from build123d import *

# Parameters (mm, degrees)
SKETCH_2_W      = 30
SKETCH_2_H      = 30
EXTRUDE_1_DEPTH = 113
EXTRUDE_2_DEPTH = 15
SKETCH_4_W      = 30
SKETCH_4_H      = 20
EXTRUDE_4_DEPTH = 3


with BuildPart() as part:
    # 草图2 → 凸台-拉伸1 (new body)
    with BuildSketch(Plane(origin=(0, 0, 0), x_dir=(1, 0, 0), z_dir=(0, 1, 0))):
        with Locations((15, 15)):
            Rectangle(SKETCH_2_W, SKETCH_2_H)
    extrude(amount=EXTRUDE_1_DEPTH)

    # 草图3 → 凸台-拉伸2 (add)
    with BuildSketch(Plane.ZY):
        with BuildLine():
            Line((-30, 113), (-24.666190379, 113))
            ThreePointArc((-24.666190379, 113), (-25.206716397, 113.665063392), (-25.4, 114.5))
            Line((-25.4, 114.5), (-25.4, 119.8))
            Line((-25.4, 119.8), (-24.9, 119.8))
            Line((-24.9, 119.8), (-24.9, 120.3))
            Line((-24.9, 120.3), (-23.1, 120.3))
            Line((-23.1, 120.3), (-23.1, 117.9))
            Line((-23.1, 117.9), (-21.815685425, 117.9))
            Line((-21.815685425, 117.9), (-19.3, 120.415685425))
            Line((-19.3, 120.415685425), (-19.3, 125.584314575))
            Line((-19.3, 125.584314575), (-21.815685425, 128.1))
            Line((-21.815685425, 128.1), (-23.1, 128.1))
            Line((-23.1, 128.1), (-23.1, 125.7))
            Line((-23.1, 125.7), (-24.9, 125.7))
            Line((-24.9, 125.7), (-24.9, 126.2))
            Line((-24.9, 126.2), (-25.4, 126.2))
            Line((-25.4, 126.2), (-25.4, 131.5))
            ThreePointArc((-25.4, 131.5), (-25.206716397, 132.334936608), (-24.666190379, 133))
            Line((-24.666190379, 133), (-30, 133))
            Line((-30, 133), (-30, 113))
        make_face()
        Polygon((-18.2, 113.1), (-18.2, 113), (-11.8, 113), (-11.8, 113.1), (-12.3, 113.1), (-12.3, 114.9), (-9.9, 114.9), (-9.9, 116.184314575), (-12.415685425, 118.7), (-17.584314575, 118.7), (-20.1, 116.184314575), (-20.1, 114.9), (-17.7, 114.9), (-17.7, 113.1), align=None)
        with BuildLine():
            ThreePointArc((-4.6, 114.5), (-4.793283603, 113.665063392), (-5.333809621, 113))
            Line((-5.333809621, 113), (0, 113))
            Line((0, 113), (0, 133))
            Line((0, 133), (-5.333809621, 133))
            ThreePointArc((-5.333809621, 133), (-4.793283603, 132.334936608), (-4.6, 131.5))
            Line((-4.6, 131.5), (-4.6, 126.2))
            Line((-4.6, 126.2), (-5.1, 126.2))
            Line((-5.1, 126.2), (-5.1, 125.7))
            Line((-5.1, 125.7), (-6.9, 125.7))
            Line((-6.9, 125.7), (-6.9, 128.1))
            Line((-6.9, 128.1), (-8.184314575, 128.1))
            Line((-8.184314575, 128.1), (-10.7, 125.584314575))
            Line((-10.7, 125.584314575), (-10.7, 120.415685425))
            Line((-10.7, 120.415685425), (-8.184314575, 117.9))
            Line((-8.184314575, 117.9), (-6.9, 117.9))
            Line((-6.9, 117.9), (-6.9, 120.3))
            Line((-6.9, 120.3), (-5.1, 120.3))
            Line((-5.1, 120.3), (-5.1, 119.8))
            Line((-5.1, 119.8), (-4.6, 119.8))
            Line((-4.6, 119.8), (-4.6, 114.5))
        make_face()
    extrude(amount=-EXTRUDE_2_DEPTH)

    # 草图4 → 凸台-拉伸4 (add)
    with BuildSketch(Plane.ZY):
        with Locations((-15, 123)):
            Rectangle(SKETCH_4_W, SKETCH_4_H)
    extrude(amount=-EXTRUDE_4_DEPTH)


solid = part.part
Input: part model. Units: mm. Frame: model coordinates. A direction names the side the tool comes from. Coordinates: 2 decimals unless noted, no trailing zeros. Loops run counter-clockwise (first coordinate to the right, second up) from the corner with the lowest first, then second, coordinate; pieces in that order, holes last.
Q1. Cut plane A-A (z = -16). Output: boundary loops of the cut face in (x, y), then the cut area to 3 significant figures.
Q2. Set-up query: faces 1 (the face through (15, 116, -15)), 2 (the face through (9, 127, -23.1)), 3 (the face through (9, 119, -23.1)). Return all of +Z, -Z, +X, -X, +Y, -Y with unobstructed straight access to the full face (end or side cutting, diameter ignored); none if empty.
Q3. Contact query for a flat-ended pin moving along its axis: pin 1 (1 mm diameter, centred on x = 6, z = -8, fed in from +Y). Output: stop coordinate, or through.
Q4. Cut plane B-B (x = 26). Output: boundary loops of the cut face in (y, z), then the cut area to 3 significant figures.
Q5. Material intervals for line 1 (Z direction, x = 10, y = 120.5); line 2 (Y direction, x = 4.5, z = -10); line 3 (Y direction, x = 9.75, z = -22.5), sorted ascending.
Q6. Draft query along Z for faces 4 (the face through (15, 123, -26)), 5 (the face through (9, 117, -4.6)), 6 (the face through (15, 66, -30)), 7 (the face through (9, 118.7, -15)). Return one class per face: +Z half, -Z half, draft (parallel to the pull), parting line (faces both ways), or undercut.
Working result:
1. outline: (0, 0) - (30, 0) - (30, 113) - (15, 113) - (15, 118.7) - (3, 118.7) - (3, 133) - (0, 133) - close
1. area: 3,520 mm2
2. face 1: +Z, -Z, +X, +Y
2. face 2: +X, +Y
2. face 3: +X
3. pin 1: stops at y = 128.1
4. outline: (0, -30) - (113, -30) - (113, 0) - (0, 0) - close
4. area: 3,390 mm2
5. line 1: z = -30 to -19.3, -10.7 to 0
5. line 2: y = 0 to 113, 114.9 to 116.28, 119.72 to 126.28
5. line 3: y = 0 to 113, 117.9 to 128.1
6. face 4: draft
6. face 5: undercut
6. face 6: -Z half
6. face 7: undercut
